```python
from build123d import *

# Parameters (mm, degrees)
SKETCH1_W             = 45.4
SKETCH1_H             = 30
BOSS_EXTRUDE1_DEPTH   = 11
SKETCH2_R             = 2.5
CUT_EXTRUDE1_DEPTH    = 30.347742673
F_3_0MM_DOWEL_HOLE1_D = 3.2
SKETCH5_R             = 3
BOSS_EXTRUDE2_DEPTH   = 4.5
SKETCH6_R             = 1.75
BOSS_EXTRUDE3_DEPTH   = 3
SKETCH7_R             = 1.5
CUT_EXTRUDE2_DEPTH    = 4


with BuildPart() as part:
    # Sketch1 → Boss-Extrude1 (new body)
    with BuildSketch(Plane(origin=(0, 0, 0), x_dir=(1, 0, 0), z_dir=(0, 1, 0))):
        Rectangle(SKETCH1_W, SKETCH1_H)
    extrude(amount=BOSS_EXTRUDE1_DEPTH)

    # Sketch2 → Cut-Extrude1 (cut, through all)
    with BuildSketch(Plane(origin=(0, 11, 0), x_dir=(1, 0, 0), z_dir=(0, 1, 0))):
        with Locations(Location((-9.5, 0, 0), (0, 0, 270))):
            Circle(SKETCH2_R)
        with Locations(Location((9.5, 0, 0), (0, 0, 270))):
            Circle(SKETCH2_R)
    extrude(amount=-CUT_EXTRUDE1_DEPTH, mode=Mode.SUBTRACT)

    # Ø3.0mm Dowel Hole1 (through all)
    with Locations(Plane(origin=(0, 11, 0), x_dir=(1, 0, 0), z_dir=(0, 1, 0))):
        with Locations((-10, 10), (10, 10), (10, -10), (-10, -10)):
            Hole(F_3_0MM_DOWEL_HOLE1_D / 2)

    # Sketch5 → Boss-Extrude2 (add)
    with BuildSketch(Plane.XZ):
        with Locations(Location((0, -5, 0), (0, 0, 270))):
            Circle(SKETCH5_R)
    extrude(amount=BOSS_EXTRUDE2_DEPTH)

    # Sketch6 → Boss-Extrude3 (add)
    with BuildSketch(Plane.XZ.offset(4.5)):
        with Locations(Location((0, -5, 0), (0, 0, 270))):
            Circle(SKETCH6_R)
    extrude(amount=BOSS_EXTRUDE3_DEPTH)

    # Sketch7 → Cut-Extrude2 (cut)
    with BuildSketch(Plane(origin=(0, 11, 0), x_dir=(1, 0, 0), z_dir=(0, 1, 0))):
        with Locations(Location((-19.7, 12, 0), (0, 0, 270))):
            Circle(SKETCH7_R)
        with Locations(Location((19.7, 12, 0), (0, 0, 270))):
            Circle(SKETCH7_R)
        with Locations(Location((19.7, -12, 0), (0, 0, 270))):
            Circle(SKETCH7_R)
        with Locations(Location((-19.7, -12, 0), (0, 0, 270))):
            Circle(SKETCH7_R)
    extrude(amount=-CUT_EXTRUDE2_DEPTH, mode=Mode.SUBTRACT)


solid = part.part
```
Verification items for the finished model (mm, model axes). A direction names the side the tool comes from. Coordinates: 2 decimals unless noted, no trailing zeros. Loops run counter-clockwise (first coordinate to the right, second up) from the corner with the lowest first, then second, coordinate; pieces in that order, holes last. Notation, with made-up numbers: (87.25, -13.5) - (137.25, -13.5) arc R18 cw to (137.25, 1.5) - close; hole circle Ø8 at (-26.75, 74). An arc over 180 degrees is marked (long way). Return JSON: item names as keys, results as strings.
1. Thickness scan on L1, parallel to X at y = 6.5, z = 10; L2, parallel to X at y = 8.6, z = 12; L3, parallel to Z at x = 9, y = 2.25. Record the ranges inside material, lowest first.
Established:
{"L1": "x = -22.7 to -11.6, -8.4 to 8.4, 11.6 to 22.7", "L2": "x = -22.7 to -21.2, -18.2 to 18.2, 21.2 to 22.7", "L3": "z = -15 to -11.25, -8.75 to -2.45, 2.45 to 8.75, 11.25 to 15"}
2. Tool access check on faces 5 (the flat face through (-20, 7, -12)), 6 (the flat face through (-2, -4.5, -5)), 7 (the cylindrical face through (11.27, 5.42, 10.97)). Record the directions out of +Z, -Z, +X, -X, +Y, -Y that give a thin tool (end or side, any length) a straight path to the whole face; none if there is none.
Established:
{"face 5": "+Y", "face 6": "-Y", "face 7": "+Y, -Y"}
3. Section check C-C, the plane x = -10. Record the boundary of the cut face in (y, z).
Established:
{"outline": "(0, -15) - (11, -15) - (11, -11.6) - (0, -11.6) - close; (0, -8.4) - (11, -8.4) - (11, -2.45) - (0, -2.45) - close; (0, 2.45) - (11, 2.45) - (11, 8.4) - (0, 8.4) - close; (0, 11.6) - (11, 11.6) - (11, 15) - (0, 15) - close"}
4. Section check B-B, the plane y = 7.5. Count the separate pieces of the cut face and the enclosed holes in it, then the cut area to 3 significant figures.
Established:
{"separate pieces": "1", "enclosed holes": "10", "area": "1,260 mm2"}
5. Mould release check, pull along X, two halves, no side actions. Record for faces 1 (the cylindrical face through (-8.73, 5.42, 10.97)), 2 (the cylindrical face through (0.08, -5.98, -3.25)), 3 (the flat face through (-22.7, 5, 0)), 4 (the flat face through (22.7, 5, 0)): +X half, -X half, draft (parallel to the pull), parting line (faces both ways), or undercut.
Established:
{"face 1": "undercut", "face 2": "parting line", "face 3": "-X half", "face 4": "+X half"}
6. Section check D-D, the plane y = 1.75. Record the boundary of the cut face in (x, z).
Established:
{"outline": "(-22.7, -15) - (22.7, -15) - (22.7, 15) - (-22.7, 15) - close; hole circle Ø5 at (-9.5, 0); hole circle Ø3.2 at (-10, -10); hole circle Ø3.2 at (-10, 10); hole circle Ø5 at (9.5, 0); hole circle Ø3.2 at (10, -10); hole circle Ø3.2 at (10, 10)"}
7. Section check A-A, the plane z = -1.5. Record the boundary of the cut face in (x, y), then the cut area to 3 significant figures.
Established:
{"outline": "(-22.7, 0) - (-11.5, 0) - (-11.5, 11) - (-22.7, 11) - close; (-7.5, 0) - (7.5, 0) - (7.5, 11) - (-7.5, 11) - close; (11.5, 0) - (22.7, 0) - (22.7, 11) - (11.5, 11) - close", "area": "411 mm2"}
8. Go/stop test with flat-tipped pins: pin 1 (0.9 mm diameter, centred on x = -19, z = -11.5, fed in from +Y); pin 2 (5 mm diameter, centred on x = -10, z = -10, fed in from -Y); pin 3 (8 mm diameter, centred on x = 4, z = 0.5, fed in from -Y); pin 4 (2.5 mm diameter, centred on x = 10, z = -10, fed in from -Y). Record where each tip stops, or that it passes through.
Established:
{"pin 1": "stops at y = 7", "pin 2": "stops at y = 0", "pin 3": "stops at y = -4.5", "pin 4": "passes through"}
